```python
from build123d import *

# Parameters (mm, degrees)
SKETCH1_R           = 2
BOSS_EXTRUDE1_DEPTH = 5


with BuildPart() as part:
    # Sketch1 → Boss-Extrude1 (new body)
    with BuildSketch(Plane.XY.offset(63)):
        with BuildLine():
            Line((13.410115914, 15.199768317), (23.030358602, 32.285219435))
            ThreePointArc((23.030358602, 32.285219435), (24.114589128, 33.843533573), (25.473776059, 35.168867371))
            ThreePointArc((25.473776059, 35.168867371), (24.928229029, 41.770329198), (19.000782012, 38.813592536))
            ThreePointArc((19.000782012, 38.813592536), (18.572370652, 36.964170331), (17.802171103, 35.229035915))
            Line((17.802171103, 35.229035915), (8.181928414, 18.143584797))
            ThreePointArc((8.181928414, 18.143584797), (7.097697889, 16.585270658), (5.738510958, 15.259936861))
            ThreePointArc((5.738510958, 15.259936861), (6.284057988, 8.658475034), (12.211505005, 11.615211695))
            ThreePointArc((12.211505005, 11.615211695), (12.639916365, 13.464633901), (13.410115914, 15.199768317))
        make_face()
        with Locations(Location((8.246602308, 12.143933367, 0), (0, 0, 180))):
            Circle(SKETCH1_R, mode=Mode.SUBTRACT)
        with Locations(Location((22.965684708, 38.284870865, 0), (0, 0, 180))):
            Circle(SKETCH1_R, mode=Mode.SUBTRACT)
    extrude(amount=-BOSS_EXTRUDE1_DEPTH)


solid = part.part
```
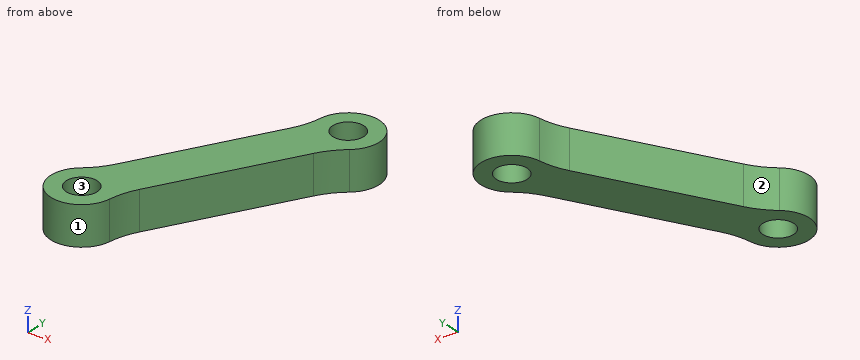
Work out the finished part from the listing and answer in its coordinate system (mm). Face numbers are marked on the shaded views. Give positions to 0.01 mm unless a question says otherwise; leave off trailing zeros. Order: outer loops, then holes, each group sorted by start corner. A loop starts at its lowest first (then second) coordinate and runs counter-clockwise, first axis right, second up. Notation, with made-up numbers: (30.5, -26.5) - (59.5, -26.5) arc R33 ccw to (59.5, 4.5) - close; hole circle Ø2 at (-27, 13.5). An arc over 180 degrees is marked (long way). One line per item, written item: value. Start each with the question number.
1. Section B-B, the plane z = 58.6 is taken. Write down the section's boundary in (x, y), then the cut area to 3 significant figures.
2. For a pull along Y with two mould halves and no side action, classify the marked faces 1, 2 and 3 as released by +Y, released by -Y, zero draft, split by the parting line, or undercut.
3. Section A-A, the plane x = 7.75 is taken. Write down the section's boundary in (y, z), then the cut area to 3 significant figures.
4. Section C-C, the plane y = 17 is taken. Write down the section's boundary in (x, z), then the cut area to 3 significant figures.
5. Each of these flat-tipped pins is pushed along its axis until it touches: pin 1 Ø1 at (x, z) = (15, 61) entering from -Y; pin 2 Ø1.5 at (y, z) = (24, 59.5) entering from -X; pin 3 Ø1 at (y, z) = (13.5, 60.5) entering from -X. Where does it stop, or does it pass through?
6. Section D-D, the plane x = 17 is taken. Write down the section's boundary in (y, z), then the cut area to 3 significant figures.
7. Consider line 1 (Y direction, x = 23, z = 59.8); line 2 (X direction, y = 37, z = 60.05); line 3 (X direction, y = 11, z = 61.8). Determine where each line is inside the solid, lowest interval first.
Filled sheet:
1. outline: (5.74, 15.26) arc R4 ccw (long way) to (12.21, 11.62) arc R10 cw to (13.41, 15.2) - (23.03, 32.29) arc R10 cw to (25.47, 35.17) arc R4 ccw (long way) to (19, 38.81) arc R10 cw to (17.8, 35.23) - (8.18, 18.14) arc R10 cw to start; hole circle Ø4 at (8.25, 12.14); hole circle Ø4 at (22.97, 38.28)
1. area: 214 mm²
2. face 1: split by the parting line
2. face 2: released by +Y
2. face 3: undercut
3. outline: (8.17, 58) - (10.21, 58) - (10.21, 63) - (8.17, 63) - close; (14.08, 58) - (17.45, 58) - (17.45, 63) - (14.08, 63) - close
3. area: 27.0 mm²
4. outline: (7.43, 58) - (14.42, 58) - (14.42, 63) - (7.43, 63) - close
4. area: 35.0 mm²
5. pin 1: y = 17.14
5. pin 2: x = 11.06
5. pin 3: x = 4.34
6. outline: (21.58, 58) - (33.8, 58) - (33.8, 63) - (21.58, 63) - close
6. area: 61.1 mm²
7. line 1: 32.23 to 36.29, 40.28 to 42.28
7. line 2: 18.58 to 21.43, 24.5 to 26.75
7. line 3: 4.41 to 6.61, 9.89 to 12.08
